```python
from build123d import *

# Parameters (mm, degrees)
SKETCH1_R           = 12.6
BOSS_EXTRUDE1_DEPTH = 29.3
SKETCH2_R           = 1.75
BOSS_EXTRUDE2_DEPTH = 11.5
SKETCH3_R           = 30
BOSS_EXTRUDE3_DEPTH = 10
SKETCH4_R           = 3
BOSS_EXTRUDE4_DEPTH = 15


with BuildPart() as part:
    # Sketch1 → Boss-Extrude1 (new body)
    with BuildSketch(Plane(origin=(0, 0, 0), x_dir=(1, 0, 0), z_dir=(0, 1, 0))):
        with Locations(Location((0, 0, 0), (0, 0, 270))):
            Circle(SKETCH1_R)
    extrude(amount=BOSS_EXTRUDE1_DEPTH)

    # Sketch2 → Boss-Extrude2 (add)
    with BuildSketch(Plane(origin=(0, 29.3, 0), x_dir=(1, 0, 0), z_dir=(0, 1, 0))):
        with Locations(Location((0, 0, 0), (0, 0, 270))):
            Circle(SKETCH2_R)
    extrude(amount=BOSS_EXTRUDE2_DEPTH)

    # Sketch3 → Boss-Extrude3 (add)
    with BuildSketch(Plane(origin=(0, 40.8, 0), x_dir=(1, 0, 0), z_dir=(0, 1, 0))):
        with Locations(Location((0, 0, 0), (0, 0, 270))):
            Circle(SKETCH3_R)
    extrude(amount=-BOSS_EXTRUDE3_DEPTH)

    # Sketch4 → Boss-Extrude4 (add)
    with BuildSketch(Plane.XZ):
        with Locations(Location((0, 5.6, 0), (0, 0, 270))):
            Circle(SKETCH4_R)
    extrude(amount=BOSS_EXTRUDE4_DEPTH)


solid = part.part
```
Part model, mm, in its own coordinate system. A direction names the side the tool comes from. Give positions to 0.01 mm unless a question says otherwise; leave off trailing zeros. Loops run counter-clockwise (first coordinate to the right, second up) from the corner with the lowest first, then second, coordinate; pieces in that order, holes last. Notation, with made-up numbers: M 66.25,-6.75 L 100.25,-6.75 A13 ccw 100.25,1.25 Z; hole C 72.5,-20.75 d7. An arc over 180 degrees is marked long. Return JSON: item names as keys, results as strings.
1) Drill centre lines: line 1 (Y direction, x = 11.5, z = 4.5); line 2 (Y direction, x = -13.5, z = 4); line 3 (X direction, y = 12, z = 11). Where is each one in solid material? Low to high.
Calculated:
{"line 1": "y = 0 to 29.3, 30.8 to 40.8", "line 2": "y = 30.8 to 40.8", "line 3": "x = -6.14 to 6.14"}
2) Flat gauge pins, fed straight in: pin 1 Ø12 at (x, y) = (-23.5, 19.5) entering from +Z; pin 2 Ø5 at (x, y) = (1.5, 4.5) entering from +Z. Where does each tip first touch, or does it go through?
Calculated:
{"pin 1": "passes through", "pin 2": "stops at z = 12.6"}
3) Saw through at D-D, the plane x = 24. List the corners of the cut face in (y, z), then the cut area to 3 significant figures.
Calculated:
{"outline": "M 30.8,-18 L 40.8,-18 L 40.8,18 L 30.8,18 Z", "area": "360 mm2"}
4) Saw through at C-C, the plane z = -10. List the corners of the cut face in (x, y), then the cut area to 3 significant figures.
Calculated:
{"outline": "M -28.28,30.8 L 28.28,30.8 L 28.28,40.8 L -28.28,40.8 Z; M -7.67,0 L 7.67,0 L 7.67,29.3 L -7.67,29.3 Z", "area": "1,010 mm2"}
5) 3-axis set-ups, long thin cutter, end or side, ignore diameter. For faces 1 (the face through (1.32, 35.87, -29.97)), 2 (the face through (-7.667, 14.445, -9.999)): which of +Z, -Z, +X, -X, +Y, -Y reach the whole face in a straight line?
Calculated:
{"face 1": "+Y, -Y", "face 2": "-Y"}
6) Pull direction Y, two halves, no side cores. Call faces 3 (the face through (0, 0, 0)), 4 (the face through (0, 40.8, 0)), 5 (the face through (-1.71, 30.04, -0.38)): released by +Y, released by -Y, zero draft, split by the parting line, or undercut.
Calculated:
{"face 3": "released by -Y", "face 4": "released by +Y", "face 5": "undercut"}
7) Saw through at A-A, the plane x = 0. List the corners of the cut face in (y, z).
Calculated:
{"outline": "M -15,2.6 L 0,2.6 L 0,-12.6 L 29.3,-12.6 L 29.3,-1.75 L 30.8,-1.75 L 30.8,-30 L 40.8,-30 L 40.8,30 L 30.8,30 L 30.8,1.75 L 29.3,1.75 L 29.3,12.6 L 0,12.6 L 0,8.6 L -15,8.6 Z"}
8) Saw through at B-B, the plane z = 0. List the corners of the cut face in (x, y), then the cut area to 3 significant figures.
Calculated:
{"outline": "M -30,30.8 L -1.75,30.8 L -1.75,29.3 L -12.6,29.3 L -12.6,0 L 12.6,0 L 12.6,29.3 L 1.75,29.3 L 1.75,30.8 L 30,30.8 L 30,40.8 L -30,40.8 Z", "area": "1,340 mm2"}
